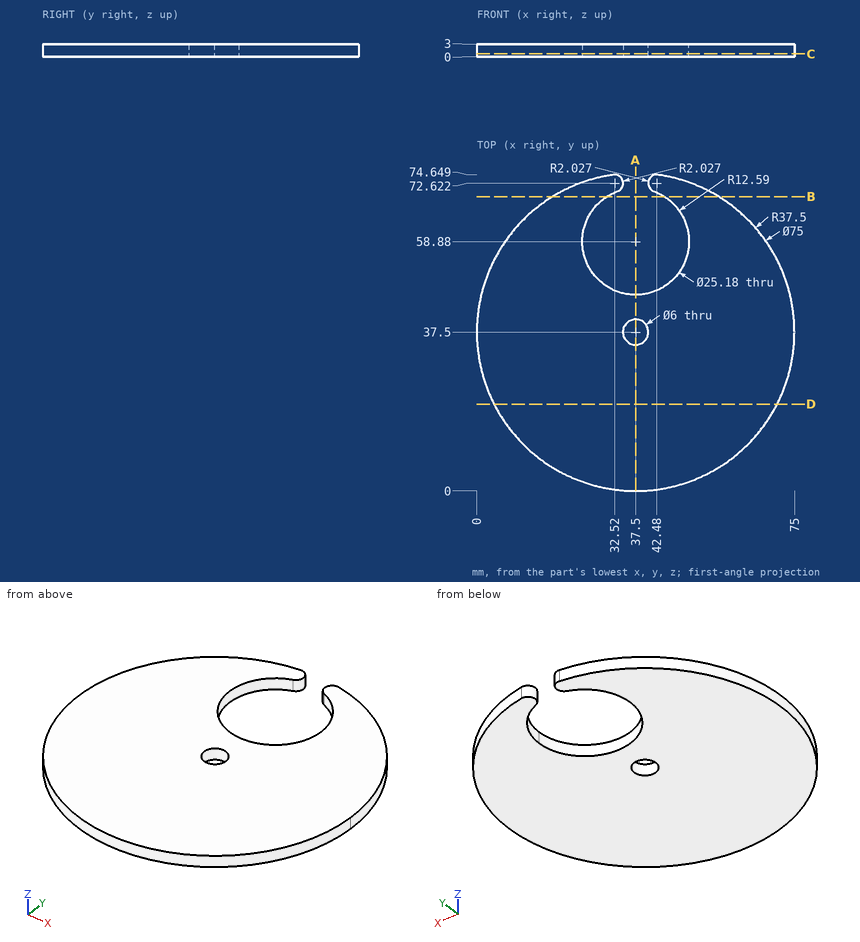
Drawing for the job (mm, zero at the part's lowest x, y, z). Round coordinates to 2 decimals unless told otherwise and drop trailing zeros. Loops run counter-clockwise (first coordinate to the right, second up) from the corner with the lowest first, then second, coordinate; pieces in that order, holes last. Notation, with made-up numbers: (85.5, -12) -> (142.5, -12) arc R12 cw to (142.5, 5) -> close; hole circle Ø1 at (-30.5, 36). An arc over 180 degrees is marked (long way). Answer in a Markdown table with one row per item.
Item 1: Pin check, flat tip, straight feed: pin 1 (5.5 mm diameter, centred on x = 37.5, y = 37.5, fed in from +Z). Stop position of the tip, or through.
Answers below:
| item | result |
|---|---|
| pin 1 | passes through |
Item 2: Saw through at B-B (y = 69.5). Write the cut outline in (x, z).
Answers below:
| item | result |
|---|---|
| outline | (17.95, 0) -> (30.74, 0) -> (30.74, 3) -> (17.95, 3) -> close; (44.26, 0) -> (57.05, 0) -> (57.05, 3) -> (44.26, 3) -> close |
Item 3: Saw through at D-D (y = 20.5). Write the cut outline in (x, z) (1 decimal).
Answers below:
| item | result |
|---|---|
| outline | (4.1, 0) -> (70.9, 0) -> (70.9, 3) -> (4.1, 3) -> close |
Item 4: Saw through at A-A (x = 37.5). Write the cut outline in (y, z).
Answers below:
| item | result |
|---|---|
| outline | (0, 0) -> (34.5, 0) -> (34.5, 3) -> (0, 3) -> close; (40.5, 0) -> (46.29, 0) -> (46.29, 3) -> (40.5, 3) -> close |
Item 5: Drill centre lines: L1, parallel to Y at x = 37.5, z = 1.4; L2, parallel to X at y = 39, z = 0.55; L3, parallel to X at y = 55, z = 2.5 (1 decimal). Where is each one in solid material? Low to high. Write a range as [from, to].
Answers below:
| item | result |
|---|---|
| L1 | y = [0, 34.5], [40.5, 46.29] |
| L2 | x = [0.03, 34.9], [40.1, 74.97] |
| L3 | x = [4.3, 25.5], [49.5, 70.7] |
Item 6: Saw through at C-C (z = 0.65). Write the cut outline in (x, y) (1 decimal), and give its area (3 significant figures).
Answers below:
| item | result |
|---|---|
| outline | (32.2, 74.6) arc R37.5 ccw (long way) to (75, 37.5) arc R37.5 ccw to (42.8, 74.6) arc R2 ccw to (41.8, 70.7) arc R12.6 cw to (50.1, 58.9) arc R12.6 cw (long way) to (33.2, 70.7) arc R2 ccw to start; hole circle Ø6 at (37.5, 37.5) |
| area | 3,870 mm² |
